Part model, mm, in its own coordinate system. Face numbers are marked on the shaded views. A direction names the side the tool comes from. Give positions to 0.01 mm unless a question says otherwise; leave off trailing zeros. Order: outer loops, then holes, each group sorted by start corner. A loop starts at its lowest first (then second) coordinate and runs counter-clockwise, first axis right, second up. Notation, with made-up numbers: (64.5, 84.25) - (79.5, 84.25) arc R34 ccw to (79.5, 123.25) - close; hole circle Ø8 at (7.5, 63). An arc over 180 degrees is marked (long way). One line per item, written item: value.
```python
from build123d import *

# Parameters (mm, degrees)
SKETCH1_W               = 20
SKETCH1_H               = 30
BOSS_EXTRUDE1_DEPTH     = 3
SKETCH2_W               = 5
SKETCH2_H               = 12
BOSS_EXTRUDE2_DEPTH     = 3
SKETCH3_R               = 7
SKETCH3_R_2             = 4
BOSS_EXTRUDE3_DEPTH     = 7
SKETCH4_R               = 4
BOSS_EXTRUDE4_DEPTH     = 1
CUT_EXTRUDE1_DEPTH      = 20.339079606
CUT_EXTRUDE1_DEPTH_BACK = 20.339079606
SKETCH5_R               = 3
SKETCH6_R               = 7
SKETCH6_R_2             = 4
BOSS_EXTRUDE6_DEPTH     = 7
SKETCH7_W               = 20
SKETCH7_H               = 3
BOSS_EXTRUDE7_DEPTH     = 19
SKETCH8_W               = 5
SKETCH8_H               = 3
BOSS_EXTRUDE8_DEPTH     = 12


with BuildPart() as part:
    # Sketch1 → Boss-Extrude1 (new body)
    with BuildSketch(Plane(origin=(0, 0, 0), x_dir=(1, 0, 0), z_dir=(0, 1, 0))):
        Rectangle(SKETCH1_W, SKETCH1_H)
    boss_extrude1 = extrude(amount=BOSS_EXTRUDE1_DEPTH)

    # Sketch2 → Boss-Extrude2 (add)
    with BuildSketch(Plane.XZ):
        with Locations((0, -9)):
            Rectangle(SKETCH2_W, SKETCH2_H)
    boss_extrude2 = extrude(amount=BOSS_EXTRUDE2_DEPTH)

    # Sketch3 → Boss-Extrude3 (add)
    with BuildSketch(Plane(origin=(0, 3, 0), x_dir=(1, 0, 0), z_dir=(0, 1, 0))):
        with Locations(Location((0, 8, 0), (0, 0, 90))):
            Circle(SKETCH3_R)
        with Locations(Location((0, 8, 0), (0, 0, 270))):
            Circle(SKETCH3_R_2, mode=Mode.SUBTRACT)
    boss_extrude3 = extrude(amount=BOSS_EXTRUDE3_DEPTH)

    # Sketch4 → Boss-Extrude4 (add)
    with BuildSketch(Plane(origin=(0, 3, 0), x_dir=(1, 0, 0), z_dir=(0, 1, 0))):
        with Locations(Location((0, 8, 0), (0, 0, 270))):
            Circle(SKETCH4_R)
    boss_extrude4 = extrude(amount=BOSS_EXTRUDE4_DEPTH)

    # Sketch5 → Cut-Extrude1 (cut, two sides: drawn at the far end of the back side and taken through both)
    with BuildSketch(Plane(origin=(0, 3, 0), x_dir=(1, 0, 0), z_dir=(0, 1, 0)).offset(-CUT_EXTRUDE1_DEPTH_BACK)):
        with Locations(Location((0, -8.5, 0), (0, 0, 90))):
            Circle(SKETCH5_R)
    extrude(amount=CUT_EXTRUDE1_DEPTH + CUT_EXTRUDE1_DEPTH_BACK, mode=Mode.SUBTRACT)

    # Sketch6 → Boss-Extrude6 (add)
    # profile 1 of 2: a face of its own
    with BuildSketch(Plane(origin=(0, 3, 0), x_dir=(1, 0, 0), z_dir=(0, 1, 0))):
        Polygon((0, 15), (-10, 15), (-10, -1), (10, -1), (10, 15), align=None)
        with BuildLine():
            ThreePointArc((7, 8), (-4.949747468, 3.050252532), (0, 15))
            ThreePointArc((0, 15), (4.949747468, 12.949747468), (7, 8))
        make_face(mode=Mode.SUBTRACT)
    # profile 2 of 2: a face of its own
    with BuildSketch(Plane(origin=(0, 3, 0), x_dir=(1, 0, 0), z_dir=(0, 1, 0))):
        with Locations((0, 8)):
            Circle(SKETCH6_R)
        with Locations(Location((0, 8, 0), (0, 0, 270))):
            Circle(SKETCH6_R_2, mode=Mode.SUBTRACT)
    boss_extrude6 = extrude(amount=BOSS_EXTRUDE6_DEPTH)

    # Sketch7 → Boss-Extrude7 (add)
    with BuildSketch(Plane.XY.offset(15)):
        with Locations((0, 1.5)):
            Rectangle(SKETCH7_W, SKETCH7_H)
    extrude(amount=BOSS_EXTRUDE7_DEPTH)

    # Mirror3: Boss-Extrude1, Boss-Extrude2, Boss-Extrude3, Boss-Extrude4, Boss-Extrude6 across plane
    add(boss_extrude1.mirror(Plane.XY.offset(17)))
    add(boss_extrude2.mirror(Plane.XY.offset(17)))
    add(boss_extrude3.mirror(Plane.XY.offset(17)))
    add(boss_extrude4.mirror(Plane.XY.offset(17)))
    add(boss_extrude6.mirror(Plane.XY.offset(17)))

    # Sketch8 → Boss-Extrude8 (add)
    with BuildSketch(Plane(origin=(0, 0, 37), x_dir=(-1, 0, 0), z_dir=(0, 0, -1))):
        with Locations((0, -1.5)):
            Rectangle(SKETCH8_W, SKETCH8_H)
    extrude(amount=BOSS_EXTRUDE8_DEPTH)


solid = part.part
```
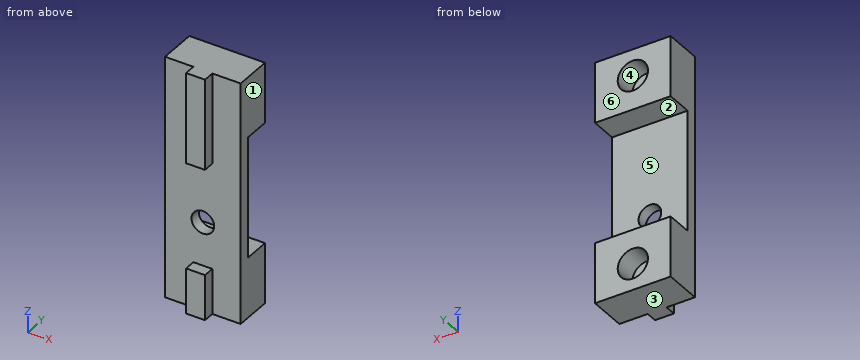
1) Slice it at A-A on y = -0.75. Write the cut outline in (x, z), then the cut area to 3 significant figures.
Answer:
outline: (-2.5, -15) - (2.5, -15) - (2.5, -3) - (-2.5, -3) - close; (-2.5, 25) - (2.5, 25) - (2.5, 49) - (-2.5, 49) - close
area: 180 mm2
2) Drop flat-ended pins along their axis: P1, Ø1.5, axis at y = -1.5, z = -10, coming from the -X side; P2, Ø8, axis at x = 0, z = 8.5, coming from the +Y side; P3, Ø4, axis at x = 1, z = 43.5, coming from the +Y side; P4, Ø2, axis at y = 6, z = 2.5, coming from the +X side. Give the stop position or say it passes through.
Answer:
P1: stops at x = -2.5
P2: stops at y = 3
P3: stops at y = 4
P4: passes through
3) Slice it at D-D on z = 8.5. Write the cut outline in (x, y), then the cut area to 3 significant figures.
Answer:
outline: (-10, 0) - (-3, 0) - (-3, 3) - (-10, 3) - close; (3, 0) - (10, 0) - (10, 3) - (3, 3) - close
area: 42.0 mm2
4) Wall check: line 1 along Z through (x, y) = (0, 3.25); line 2 along Z through (x, y) = (-0.5, -1.5); line 3 along Y through (x, z) = (2.25, 23.5). Give the ranges that are in metal, low to high. Write a range as [from, to].
Answer:
line 1: z = [-15, 1], [33, 49]
line 2: z = [-15, -3], [25, 49]
line 3: y = [0, 3]
5) Slice it at B-B on x = 0. Write the cut outline in (y, z), then the cut area to 3 significant figures.
Answer:
outline: (-3, -15) - (10, -15) - (10, -12) - (4, -12) - (4, -4) - (10, -4) - (10, 1) - (3, 1) - (3, 5.5) - (0, 5.5) - (0, -3) - (-3, -3) - close; (-3, 25) - (0, 25) - (0, 11.5) - (3, 11.5) - (3, 33) - (10, 33) - (10, 38) - (4, 38) - (4, 46) - (10, 46) - (10, 49) - (-3, 49) - close
area: 410 mm2
6) Which spindle directions (+Z, -Z, +X, -X, +Y, -Y) get a long thin tool onto all of the face, cutting with end or side? Do the marked faces 4, 5 and 6. Say none if no direction does.
Answer:
face 4: +Y
face 5: +X, -X, +Y
face 6: +Z, -Z, +X, -X, +Y
7) Two-plate mould, pull along Z, no slides. Class the marked faces 1, 2 and 3: pulls with the +Z half, pulls with the -Z half, needs draft (parallel to the pull), parting line crosses it, or undercut.
Answer:
face 1: needs draft
face 2: undercut
face 3: pulls with the -Z half
8) Slice it at C-C on y = 6. Write the cut outline in (x, z).
Answer:
outline: (-10, -15) - (10, -15) - (10, 1) - (-10, 1) - close; (-10, 33) - (10, 33) - (10, 49) - (-10, 49) - close; hole circle Ø8 at (0, -8); hole circle Ø8 at (0, 42)
